from build123d import *

# Parameters (mm, degrees)
F1_DEPTH = 110
F3_DEPTH = 69.792666


with BuildPart() as f1:
    # F0 (on Top) → F1 (new body)
    with BuildSketch(Plane.XY):
        with BuildLine():
            ThreePointArc((-34.895833, -15), (-33.431367, -18.535534), (-29.895833, -20))
            Line((-29.895833, -20), (29.895833, -20))
            ThreePointArc((29.895833, -20), (33.431367, -18.535534), (34.895833, -15))
            Line((34.895833, -15), (34.895833, 15))
            ThreePointArc((34.895833, 15), (33.431367, 18.535534), (29.895833, 20))
            Line((29.895833, 20), (-29.895833, 20))
            ThreePointArc((-29.895833, 20), (-33.431367, 18.535534), (-34.895833, 15))
            Line((-34.895833, 15), (-34.895833, -15))
        make_face()
    extrude(amount=F1_DEPTH)

    # F2 (on face) → F3 (cut, through all)
    with BuildSketch(Plane(origin=(-34.895833, 0, 0), x_dir=(0, -1, 0), z_dir=(-1, 0, 0))):
        Polygon((-20.880114, 110), (-20.880114, 104.359761), (10.082219, 110), align=None)
    extrude(amount=-F3_DEPTH, mode=Mode.SUBTRACT)


solid = f1.part
Part model, mm, in its own coordinate system. Round coordinates to 2 decimals unless told otherwise and drop trailing zeros. Order: outer loops, then holes, each group sorted by start corner. A loop starts at its lowest first (then second) coordinate and runs counter-clockwise, first axis right, second up. Notation, with made-up numbers: (28.5, 73) -> (43.5, 73) arc R27 ccw to (43.5, 99) -> close; hole circle Ø3 at (-33.75, 36.5). An arc over 180 degrees is marked (long way). Put each result on its own line as item: value.
Q1. Band-saw the part on B-B (y = 0). Give the cut face in (x, z), and give its area (3 significant figures).
From the geometry:
outline: (-34.9, 0) -> (34.9, 0) -> (34.9, 108.16) -> (-34.9, 108.16) -> close
area: 7,550 mm2
Q2. Wall check: line 1 (X direction, y = 15.5, z = 18.5); line 2 (Y direction, x = -30, z = 29); line 3 (Z direction, x = -17.5, y = -1). Give the ranges that are in metal, low to high. Write a range as [from, to].
From the geometry:
line 1: x = [-34.87, 34.87]
line 2: y = [-20, 20]
line 3: z = [0, 108.35]
Q3. Pull direction Z, two halves, no side cores. Call faces 1 (the face through (0, -20, 54)), 2 (the face through (-0.49, 5.17, 107.22)), 3 (the face through (0, 0, 0)): pulls with the +Z half, pulls with the -Z half, needs draft (parallel to the pull), parting line crosses it, or undercut.
From the geometry:
face 1: needs draft
face 2: pulls with the +Z half
face 3: pulls with the -Z half
Q4. Band-saw the part on A-A (x = -17). Give the cut face in (y, z), and give its area (3 significant figures).
From the geometry:
outline: (-20, 0) -> (20, 0) -> (20, 104.52) -> (-10.08, 110) -> (-20, 110) -> close
area: 4,320 mm2
